from build123d import *

# Parameters (mm, degrees)
SKETCH_1_R      = 50
SKETCH_1_R_2    = 35
EXTRUDE_1_DEPTH = 96
CHAMFER_1_SIZE  = 1


with BuildPart() as part:
    # 草图1 → 凸台-拉伸1 (new body)
    with BuildSketch(Plane(origin=(0, 0, 0), x_dir=(0, 0, -1), z_dir=(1, 0, 0))):
        Circle(SKETCH_1_R)
        Circle(SKETCH_1_R_2, mode=Mode.SUBTRACT)
    extrude(amount=EXTRUDE_1_DEPTH)

    # 倒角1
    chamfer_1_edges = [part.edges().sort_by_distance(p)[0] for p in [
        (0, 0, 50),
        (96, 0, 50),
        (0, 0, 35),
        (96, 0, 35),
    ]]
    chamfer(chamfer_1_edges, length=CHAMFER_1_SIZE)


solid = part.part
Read the model definition and answer for the solid it produces. Units are mm, in the model's axes. Give positions to 0.01 mm unless a question says otherwise; leave off trailing zeros. Write each loop counter-clockwise with the first axis right and the second up, starting at its lowest first coordinate (ties: lowest second). Pieces come first, ordered by that corner, then holes. Notation, with made-up numbers: (3.25, 88.5) -> (45.25, 88.5) arc R23 cw to (45.25, 102.5) -> close; hole circle Ø8 at (-31.5, 83.5). An arc over 180 degrees is marked (long way). Answer as a JSON object with one key per item and string values. Group by question number.
1) Each of these flat-tipped pins is pushed along its axis until it touches: P1, Ø2, axis at x = 48, z = 19.5, coming from the +Y side; P2, Ø2, axis at x = 24.5, y = 17, coming from the +Z side; P3, Ø8, axis at x = 12.5, z = -29.5, coming from the +Y side. Where does it stop, or does it pass through?
2) Consider L1, parallel to Y at x = 22, z = 0; L2, parallel to Z at x = 52, y = -30.5; L3, parallel to Y at x = 35.5, z = -20. Determine where each line is inside the solid, lowest interval first. Write a range as from..to.
3) Find section C-C (x = 90). Write down the section's boundary in (y, z).
4) Find section A-A (z = 0). Write down the section's boundary in (x, y).
5) The mould has two halves that part along Z. Classify faces 1 (the cylindrical face through (47.34, 15.02, -47.69)), 2 (the cylindrical face through (47, -21, 28)), 3 (the flat face through (0, 26, 26)): +Z half, -Z half, draft (parallel to the pull), parting line (faces both ways), or undercut.
Values follow:
{
 "1": {"P1": "stops at y = 46.45", "P2": "stops at z = 47.37", "P3": "stops at y = 43.01"},
 "2": {"L1": "y = -50..-35, 35..50", "L2": "z = -39.62..-17.17, 17.17..39.62", "L3": "y = -45.83..-28.72, 28.72..45.83"},
 "3": {"outline": "circle Ø100 at (0, 0); hole circle Ø70 at (0, 0)"},
 "4": {"outline": "(0, -49) -> (1, -50) -> (95, -50) -> (96, -49) -> (96, -36) -> (95, -35) -> (1, -35) -> (0, -36) -> close; (0, 36) -> (1, 35) -> (95, 35) -> (96, 36) -> (96, 49) -> (95, 50) -> (1, 50) -> (0, 49) -> close"},
 "5": {"face 1": "parting line", "face 2": "undercut", "face 3": "draft"}
}
